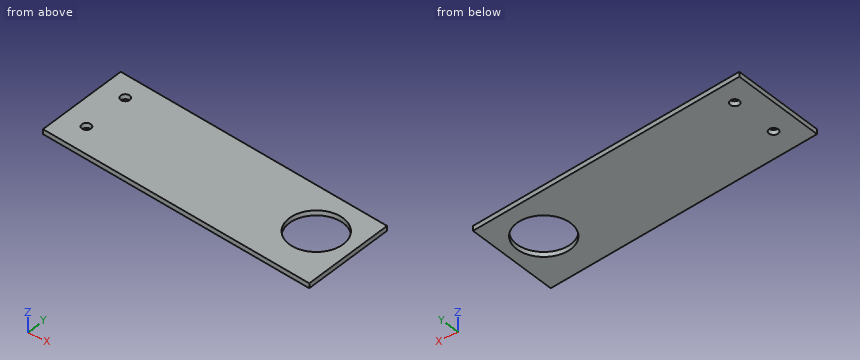
Autodesk Inventor part; units mm, degrees
ref_plane "YZ Plane" through (0, 0, 0) normal (1, 0, 0) x (0, 1, 0)
ref_plane "XZ Plane" through (0, 0, 0) normal (0, 1, 0) x (-1, 0, 0)
ref_plane "XY Plane" through (0, 0, 0) normal (0, 0, 1) x (1, 0, 0)
sketch "Sketch1" plane through (0, 0, 0) normal (0, 0, 1) x (1, 0, 0)
  line L0 (0, 0) -> (151.8201, -13.2825)
  line L1 (151.8201, -13.2825) -> (151.8201, 37.5175)
  line L2 (151.8201, 37.5175) -> (0, 50.8)
  line L3 (0, 50.8) -> (0, 0)
  dimension "d0" = 50.8
  dimension "d1" = 50.8
  dimension "d2" = 85
  dimension "d3" = 152.4
extrude "Extrusion1" add sketch "Sketch1" along normal blind 2.54
hole "Hole1" at (131.5001, 16.3479, 2.54) direction (0, 0, -1) diameter 28.575 end through all
sketch "Sketch2" plane through (0, 0, 0) normal (0, 0, -1) x (-1, 0, 0)
  line L0 (0, 0) -> (-151.8201, -13.2825)
  line L1 (0, 0) -> (-33.0355, 0)
  line L2 (0, 50.8) -> (0, 0)
  point P0 (-12.7, 38.1)
  point P1 (-12.7, 12.7)
  dimension "d15" = 12.7
  dimension "d16" = 38.1
  dimension "d17" = 12.7
  dimension "d18" = 12.7
hole "Hole2" at (12.7, 38.1, 0) at (12.7, 12.7, 0) direction (0, 0, 1) diameter 4.8514 end through all
properties part number "CAR_050_Sweeper Bar arms"
Check sheet for the modelled part. Datum: model origin and axes. Units: mm. Round coordinates to 2 decimals unless told otherwise and drop trailing zeros. Loops run counter-clockwise (first coordinate to the right, second up) from the corner with the lowest first, then second, coordinate; pieces in that order, holes last. Notation, with made-up numbers: M -35.5,71.5 L 0.5,71.5 A20 ccw 0.5,95.5 Z; hole C 63.25,14 d9. An arc over 180 degrees is marked long. One line per question, with ' | ' between items. Start each with the question number.
Item 1: Scan lines: probe 1 along Y at (x, z) = (12.7, 1.8); probe 2 along X at (y, z) = (12.7, 1.3); probe 3 along X at (y, z) = (12, 1). Record each from-to range of solid material in increasing order.
Item 2: Section check A-A (y = 4). Record the boundary of the cut face in (x, z), and give its area (3 significant figures).
Item 3: Section check D-D (y = 12.7). Record the boundary of the cut face in (x, z).
Item 4: Section check B-B (x = 12.7). Record the boundary of the cut face in (y, z), and give its area (3 significant figures).
Item 5: Gauge pin test, flat end, axial feed: pin 1 Ø1.5 at (x, z) = (122.5, 1.5) entering from -Y. Record the tip position at first contact, or that the pin passes through.
Item 6: Section check C-C (x = 127). Record the boundary of the cut face in (y, z).
Worked out:
1) probe 1: -1.11 to 10.27, 15.13 to 35.67, 40.53 to 49.69 | probe 2: 0 to 10.27, 15.13 to 117.69, 145.31 to 151.82 | probe 3: 0 to 10.38, 15.02 to 117.89, 145.11 to 151.82
2) outline: M 0,0 L 124.31,0 L 124.31,2.54 L 0,2.54 Z; M 138.69,0 L 151.82,0 L 151.82,2.54 L 138.69,2.54 Z | area: 349 mm^2
3) outline: M 0,0 L 10.27,0 L 10.27,2.54 L 0,2.54 Z; M 15.13,0 L 117.69,0 L 117.69,2.54 L 15.13,2.54 Z; M 145.31,0 L 151.82,0 L 151.82,2.54 L 145.31,2.54 Z
4) outline: M -1.11,0 L 10.27,0 L 10.27,2.54 L -1.11,2.54 Z; M 15.13,0 L 35.67,0 L 35.67,2.54 L 15.13,2.54 Z; M 40.53,0 L 49.69,0 L 49.69,2.54 L 40.53,2.54 Z | area: 104 mm^2
5) pin 1: y = -10.78
6) outline: M -11.11,0 L 2.79,0 L 2.79,2.54 L -11.11,2.54 Z; M 29.91,0 L 39.69,0 L 39.69,2.54 L 29.91,2.54 Z
